Part model, mm, in its own coordinate system. Face numbers are marked on the shaded views. A direction names the side the tool comes from. Coordinates: 2 decimals unless noted, no trailing zeros. Write each loop counter-clockwise with the first axis right and the second up, starting at its lowest first coordinate (ties: lowest second). Pieces come first, ordered by that corner, then holes. Notation, with made-up numbers: (-2.75, -25) -> (18.25, -25) arc R9 ccw to (18.25, -21) -> close; hole circle Ø8 at (38, 12). An arc over 180 degrees is marked (long way). Write item = value, one per line.
from build123d import *

# Parameters (mm, degrees)
EXTRUDE1_DEPTH     = 139.7
SKETCH2_R          = 2.3876
CUT_EXTRUDE1_DEPTH = 2.539999999
SKETCH3_R          = 2.3876
CUT_EXTRUDE2_DEPTH = 2.54
SKETCH4_R          = 3.81
CUT_EXTRUDE3_DEPTH = 2.539999999
SKETCH5_R          = 7.1755
SKETCH5_R_2        = 3.81
EXTRUDE2_DEPTH     = 6.985
FILLET1_R          = 2.54
FILLET2_R          = 5.08


with BuildPart() as part:
    # Sketch1 → Extrude1 (new body)
    with BuildSketch(Plane.XY):
        Polygon((5980.833305588, -6626.860000001), (6002.006203139, -6626.860000001), (6002.006203139, -6629.4), (5979.781203139, -6629.4), (5951.206203139, -6600.825), (5951.206203139, -6578.6), (5953.746203139, -6578.6), (5953.746203139, -6599.772897553), (5967.289754364, -6613.316448778), align=None)
    extrude(amount=EXTRUDE1_DEPTH)

    # Sketch2 → Cut-Extrude1 (cut)
    with BuildSketch(Plane.XZ.offset(6629.4)):
        with Locations(Location((5990.881003139, 127, 0), (0, 0, 270))):
            Circle(SKETCH2_R)
        with Locations(Location((5990.881003139, 69.85, 0), (0, 0, 270))):
            Circle(SKETCH2_R)
        with Locations(Location((5990.881003139, 12.7, 0), (0, 0, 270))):
            Circle(SKETCH2_R)
    extrude(amount=-CUT_EXTRUDE1_DEPTH, mode=Mode.SUBTRACT)

    # Sketch3 → Cut-Extrude2 (cut)
    with BuildSketch(Plane.ZY.offset(-5951.206203139)):
        with Locations((127, -6589.7252)):
            Circle(SKETCH3_R)
        with Locations((69.85, -6589.7252)):
            Circle(SKETCH3_R)
        with Locations((12.7, -6589.7252)):
            Circle(SKETCH3_R)
    extrude(amount=-CUT_EXTRUDE2_DEPTH, mode=Mode.SUBTRACT)

    # Sketch4 → Cut-Extrude3 (cut)
    with BuildSketch(Plane(origin=(-324.80939843, -324.80939843, 0), x_dir=(0, 0, 1), z_dir=(-0.7071067811865477, -0.7071067811865475, 0))):
        with Locations(Location((69.85, -8895.831957677, 0), (0, 0, 270))):
            Circle(SKETCH4_R)
        with Locations(Location((12.7, -8895.831957677, 0), (0, 0, 270))):
            Circle(SKETCH4_R)
    extrude(amount=-CUT_EXTRUDE3_DEPTH, mode=Mode.SUBTRACT)

    # Sketch5 → Extrude2 (add)
    with BuildSketch(Plane(origin=(-323.013347207, -323.013347207, 0), x_dir=(0, 0, -1), z_dir=(0.7071067811865477, 0.7071067811865475, 0))):
        with Locations(Location((-69.85, -8895.831957677, 0), (0, 0, 270))):
            Circle(SKETCH5_R)
        with Locations(Location((-69.85, -8895.831957677, 0), (0, 0, 270))):
            Circle(SKETCH5_R_2, mode=Mode.SUBTRACT)
        with Locations(Location((-12.7, -8895.831957677, 0), (0, 0, 270))):
            Circle(SKETCH5_R)
        with Locations(Location((-12.7, -8895.831957677, 0), (0, 0, 270))):
            Circle(SKETCH5_R_2, mode=Mode.SUBTRACT)
    extrude(amount=EXTRUDE2_DEPTH)

    # Fillet1
    fillet1_edges = [part.edges().sort_by_distance(p)[0] for p in [
        (5980.833305588, -6626.860000001, 69.85),
        (5953.746203139, -6599.772897553, 69.85),
    ]]
    fillet(fillet1_edges, radius=FILLET1_R)

    # Fillet2
    fillet2_edges = [part.edges().sort_by_distance(p)[0] for p in [
        (5979.781203139, -6629.4, 69.85),
        (5951.206203139, -6600.825, 69.85),
    ]]
    fillet(fillet2_edges, radius=FILLET2_R)


solid = part.part
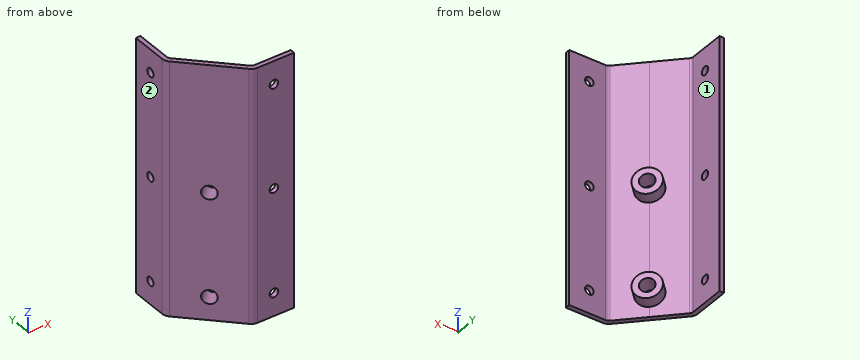
Q1. Saw through at C-C on z = 12.7. Give the cut face in (x, y).
Model answer:
outline = (5951.21, -6598.72) arc R5.08 ccw to (5952.69, -6602.31) -> (5962.8, -6612.42) -> (5969.53, -6605.68) -> (5967.16, -6603.3) -> (5962.22, -6608.24) -> (5954.49, -6600.52) arc R2.54 cw to (5953.75, -6598.72) -> (5953.75, -6592.11) -> (5951.21, -6592.11) -> close; (5951.21, -6587.34) -> (5953.75, -6587.34) -> (5953.75, -6578.6) -> (5951.21, -6578.6) -> close; (5968.19, -6617.81) -> (5978.29, -6627.91) arc R5.08 ccw to (5981.89, -6629.4) -> (5988.49, -6629.4) -> (5988.49, -6626.86) -> (5981.89, -6626.86) arc R2.54 cw to (5980.09, -6626.12) -> (5972.36, -6618.39) -> (5977.3, -6613.45) -> (5974.92, -6611.07) -> close; (5993.27, -6629.4) -> (6002.01, -6629.4) -> (6002.01, -6626.86) -> (5993.27, -6626.86) -> close
Q2. Saw through at B-B on z = 53.5. Give the cut face in (x, y), and give its area (3 significant figures).
Model answer:
outline = (5951.21, -6598.72) arc R5.08 ccw to (5952.69, -6602.31) -> (5978.29, -6627.91) arc R5.08 ccw to (5981.89, -6629.4) -> (6002.01, -6629.4) -> (6002.01, -6626.86) -> (5981.89, -6626.86) arc R2.54 cw to (5980.09, -6626.12) -> (5954.49, -6600.52) arc R2.54 cw to (5953.75, -6598.72) -> (5953.75, -6578.6) -> (5951.21, -6578.6) -> close
area = 209 mm²
Q3. Saw through at D-D on x = 5960. Give the cut face in (y, z), and give its area (3 significant figures).
Model answer:
outline = (-6609.62, 0) -> (-6606.03, 0) -> (-6606.03, 139.7) -> (-6609.62, 139.7) -> close
area = 502 mm²
Q4. Pin check, flat tips, straight feed: pin 1 (4 mm diameter, centred on x = 5990.88, z = 127, fed in from +Y); pin 2 (16 mm diameter, centred on y = -6588, z = 60, fed in from +X); pin 3 (10 mm diameter, centred on x = 5992, z = 67.5, fed in from +Y); pin 4 (6 mm diameter, centred on y = -6619.5, z = 87, fed in from -X). Stop position of each tip, or through.
Model answer:
pin_1 = through
pin_2 = 5953.75
pin_3 = -6626.86
pin_4 = 5966.88
Q5. Probe line 1 (Y direction, x = 5997, z = 64.5); line 2 (Y direction, x = 5952, z = 69); line 3 (X direction, y = -6628.45, z = 12.7). List the from-to ranges inside material, lowest first. Write a range as from..to.
Model answer:
line_1 = -6629.4..-6626.86
line_2 = -6601.45..-6591.96, -6587.49..-6578.6
line_3 = 5978.93..5988.49, 5993.27..6002.01
Q6. Saw through at A-A on z = 127. Give the cut face in (x, y).
Model answer:
outline = (5951.21, -6598.72) arc R5.08 ccw to (5952.69, -6602.31) -> (5978.29, -6627.91) arc R5.08 ccw to (5981.89, -6629.4) -> (5988.49, -6629.4) -> (5988.49, -6626.86) -> (5981.89, -6626.86) arc R2.54 cw to (5980.09, -6626.12) -> (5954.49, -6600.52) arc R2.54 cw to (5953.75, -6598.72) -> (5953.75, -6592.11) -> (5951.21, -6592.11) -> close; (5951.21, -6587.34) -> (5953.75, -6587.34) -> (5953.75, -6578.6) -> (5951.21, -6578.6) -> close; (5993.27, -6629.4) -> (6002.01, -6629.4) -> (6002.01, -6626.86) -> (5993.27, -6626.86) -> close
Q7. Which spindle directions (+Z, -Z, +X, -X, +Y, -Y) get a long thin tool onto all of the face, cutting with end or side? Do the marked faces 1 and 2. Say none if no direction does.
Model answer:
face_1 = +Z, -Z, +X, +Y
face_2 = +Z, -Z, -X, +Y, -Y
